Input: part model. Units: mm. Frame: model coordinates. A direction names the side the tool comes from. Round coordinates to 2 decimals unless told otherwise and drop trailing zeros. Loops run counter-clockwise (first coordinate to the right, second up) from the corner with the lowest first, then second, coordinate; pieces in that order, holes last.
(1) Cut plane D-D, the plane x = -41.5. Output: boundary loops of the cut face in (y, z).
(2) Line query: line 1 (Y direction, x = 0, z = 18); line 2 (X direction, y = -11, z = 29.5) (3 decimals); line 3 (Y direction, x = 45, z = 45). Output: solid intervals per line, ascending.
(3) Cut plane C-C, the plane z = 29. Output: boundary loops of the cut face in (x, y), and give its area (3 significant figures).
(4) Cut plane A-A, the plane x = -8. Output: boundary loops of the cut face in (y, z), and give its area (3 significant figures).
(5) Cut plane B-B, the plane y = -36. Output: boundary loops of the cut face in (x, z), and give its area (3 significant figures).
(6) Access query for faces 1 (the face through (158.95, -4, 8)), 2 (the face through (134, -11, -17)), 3 (the face through (-55, 1, -50)). Directions: +Z, -Z, +X, -X, +Y, -Y. A direction counts if a zero-diameter tool reaches every point of the face in a straight line with its end or side. Return the directions, or none.
(7) First-contact query: pin 1 Ø12 at (x, z) = (165.5, 6.5) entering from -Y; pin 2 Ø1 at (x, z) = (107.5, 25.5) entering from -Y; pin 3 Ø1.5 at (x, z) = (3.5, -10.5) entering from -Y. Flat tips, straight axial feed; report the tip coordinate or a pass-through.
from build123d import *

# Parameters (mm, degrees)
SKETCH1_R           = 50
BOSS_EXTRUDE1_DEPTH = 50
BOSS_EXTRUDE2_REACH = 202
SKETCH2_R           = 45


with BuildPart() as part:
    # Sketch1 → Boss-Extrude1 (new body, symmetric)
    with BuildSketch(Plane.XY):
        with BuildLine():
            Line((-80, -40), (-80, 40))
            Line((-80, 40), (-19.421277332, 62.030750332))
            ThreePointArc((-19.421277332, 62.030750332), (64.982457362, -1.51004478), (-22.281665693, -61.061668614))
            Line((-22.281665693, -61.061668614), (-80, -40))
        make_face()
        Circle(SKETCH1_R, mode=Mode.SUBTRACT)
    extrude(amount=BOSS_EXTRUDE1_DEPTH, both=True)

    # Sketch2 → Boss-Extrude2 (add, up to next)
    with BuildSketch(Plane(origin=(120, 0, 0), x_dir=(0, 0, -1), z_dir=(1, 0, 0)), mode=Mode.PRIVATE) as boss_extrude2_sk1:
        Circle(SKETCH2_R)
    boss_extrude2_tool1 = extrude(boss_extrude2_sk1.sketch, amount=-BOSS_EXTRUDE2_REACH, mode=Mode.PRIVATE) - part.part
    add(boss_extrude2_tool1.solids().sort_by_distance((120, 0, 0))[0])

    # Sketch3 → Revolve1 (revolve)
    with BuildSketch(Plane.XY):
        Polygon((120, 0), (120, -20), (134, -20), (134, -25), (149, -25), (149, -19.298257311), (158.95018422, -18.301345082), (158.95018422, -8.331313354), (195, 0), align=None)
    revolve(axis=Axis((0, 0, 0), (1, 0, 0)))


solid = part.part
Reported:
1. outline: (-54.05, -50) - (-27.89, -50) - (-27.89, 50) - (-54.05, 50) - close; (27.89, -50) - (54, -50) - (54, 50) - (27.89, 50) - close
2. line 1: y = -65 to -50, 50 to 65
2. line 2: x = -80 to -48.775, 48.775 to 120
2. line 3: y = -46.9 to -21.79, 21.79 to 46.9
3. outline: (-80, -40) - (-22.28, -61.06) arc R65 ccw to (55.15, -34.41) - (120, -34.41) - (120, 34.41) - (55.15, 34.41) arc R65 ccw to (-19.42, 62.03) - (-80, 40) - close; hole circle Ø100 at (0, 0)
3. area: 11,500 mm2
4. outline: (-64.51, -50) - (-49.36, -50) - (-49.36, 50) - (-64.51, 50) - close; (49.36, -50) - (64.51, -50) - (64.51, 50) - (49.36, 50) - close
4. area: 3,030 mm2
5. outline: (-80, -50) - (-34.7, -50) - (-34.7, 50) - (-80, 50) - close; (34.7, -50) - (54.12, -50) - (54.12, -27) - (120, -27) - (120, 27) - (54.12, 27) - (54.12, 50) - (34.7, 50) - close
5. area: 10,000 mm2
6. face 1: +X
6. face 2: none
6. face 3: -Z, +X, -X, +Y, -Y
7. pin 1: stops at y = -7.47
7. pin 2: stops at y = -37.42
7. pin 3: stops at y = -64.94
